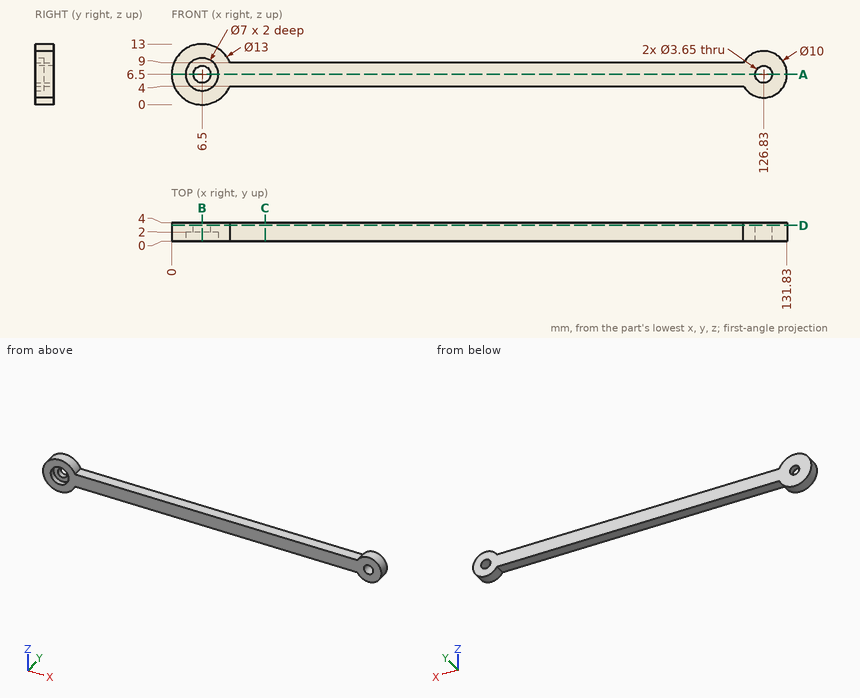
Study the drawing (mm; zero at the part's minimum x, y, z) and answer. Give positions to 0.01 mm unless a question says otherwise; leave off trailing zeros. Write each loop counter-clockwise with the first axis right and the second up, starting at its lowest first coordinate (ties: lowest second). Pieces come first, ordered by that corner, then holes. Notation, with made-up numbers: (7, -31) -> (52, -31) arc R16 ccw to (52, -18) -> close; hole circle Ø11 at (-7, 42). An arc over 180 degrees is marked (long way). Answer as a JSON object with one key per item and string values. Group by question number.
1) Find section C-C (x = 20). Write down the section's boundary in (y, z).
2) Consider L1, parallel to X at y = 0.8, z = 7.75; L2, parallel to Y at x = 6.5, z = 4.25; L3, parallel to Z at x = 106.5, y = 1.65. Determine where each line is inside the solid, lowest interval first. Write a range as from..to.
3) Find section B-B (x = 6.5). Write down the section's boundary in (y, z) (3 decimals), and give its area (3 significant figures).
4) Find section D-D (y = 3.4). Write down the section's boundary in (x, z) (3 decimals).
5) Each of these flat-tipped pins is pushed along its axis until it touches: P1, Ø2, axis at x = 43, y = 1.5, coming from the -Z side; P2, Ø4, axis at x = 6.5, z = 6.5, coming from the +Y side; P3, Ø6.5, axis at x = 6.5, z = 6.5, coming from the -Y side. Where does it stop, or does it pass through?
6) Find section A-A (z = 6.5). Write down the section's boundary in (x, y) (3 decimals), and give its area (3 significant figures).
Values follow:
{
 "1": {"outline": "(0, 4) -> (4, 4) -> (4, 9) -> (0, 9) -> close"},
 "2": {"L1": "x = 0.12..3.23, 9.77..125.5, 128.16..131.67", "L2": "y = 2..4", "L3": "z = 4..9"},
 "3": {"outline": "(0, 0) -> (4, 0) -> (4, 4.675) -> (2, 4.675) -> (2, 3) -> (0, 3) -> close; (0, 10) -> (2, 10) -> (2, 8.325) -> (4, 8.325) -> (4, 13) -> (0, 13) -> close", "area": "30.7 mm2"},
 "4": {"outline": "(12.5, 4) -> (122.5, 4) arc R5 ccw (long way) to (122.5, 9) -> (12.5, 9) arc R6.5 ccw (long way) to start; hole circle Ø3.65 at (6.5, 6.5); hole circle Ø3.65 at (126.83, 6.5)"},
 "5": {"P1": "stops at z = 4", "P2": "stops at y = 4", "P3": "stops at y = 2"},
 "6": {"outline": "(0, 0) -> (3, 0) -> (3, 2) -> (4.675, 2) -> (4.675, 4) -> (0, 4) -> close; (8.325, 2) -> (10, 2) -> (10, 0) -> (125.005, 0) -> (125.005, 4) -> (8.325, 4) -> close; (128.655, 0) -> (131.83, 0) -> (131.83, 4) -> (128.655, 4) -> close", "area": "491 mm2"}
}
